For this review, take the finished solid that the model builds, in its own axes (mm). Face numbers are marked on the shaded views. A direction names the side the tool comes from. Coordinates: 2 decimals unless noted, no trailing zeros. Order: outer loops, then holes, each group sorted by start corner. A loop starts at its lowest first (then second) coordinate and runs counter-clockwise, first axis right, second up. Notation, with made-up numbers: (6.25, 7) -> (15.25, 7) arc R25 cw to (15.25, 24) -> close; hole circle Ø8 at (6.25, 60). An arc over 180 degrees is marked (long way). Return JSON: item names as keys, results as strings. Group by question number.
Item 1: Take a section at B-B (z = 0.5). Write out the cut boundary in (x, y).
Item 2: Machinability: for the marked faces 1, 2 and 3, which of the approach directions +Z, -Z, +X, -X, +Y, -Y give a long, thin tool a straight path to every point of the face, cutting with its end or side? Answer none if there is none.
Item 3: Insertion check: pin 1 (5 mm diameter, centred on y = -2, z = 13, fed in from +X); pin 2 (6 mm diameter, centred on x = -6.5, z = 19.5, fed in from -Y) (3 decimals); pin 3 (6 mm diameter, centred on x = 21, z = 15.5, fed in from -Y). Each pin has a flat end and moves straight along its axis. Give the tip position at first contact, or say it passes through.
Item 4: Draft analysis for pull direction Z (two halves, no side actions). For the marked faces 4, 5, 6 and 7, state which applies: +Z half, -Z half, draft (parallel to the pull), parting line (faces both ways), or undercut.
Item 5: Take a section at C-C (y = 13). Write out the cut boundary in (x, z), then the cut area to 3 significant figures.
Item 6: Take a section at A-A (x = 34.5). Write out the cut boundary in (y, z), then the cut area to 3 significant figures.
Item 7: For line 1 along Y through (x, z) = (34, 20.5); line 2 along Z through (x, y) = (12, -19); line 3 along Y through (x, z) = (2, 6.5) (3 decimals), list the stretches that pass through material, from the lowest coordinate up.
Item 8: Take a section at D-D (z = 18.5). Count the separate pieces of the cut face and the enclosed holes in it, then the cut area to 3 significant figures.
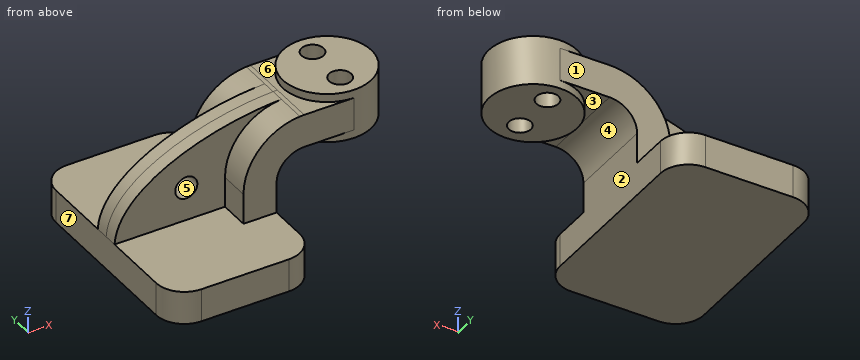
```python
from build123d import *

# Parameters (mm, degrees)
F1_DEPTH = 25
F0_W     = 10
F0_H     = 7.5
F2_DEPTH = 10
F3_DEPTH = 3.125
F5_R     = 6.35
F7_D     = 5
F9_D     = 5


with BuildPart() as f1:
    # F0 (on Front) → F1 (new body, symmetric)
    with BuildSketch(Plane.XZ):
        Polygon((8.75, 3.75), (-16.25, 3.75), (-16.25, -3.75), (16.25, -3.75), (16.25, 3.75), align=None)
    extrude(amount=F1_DEPTH, both=True)

    # F0 (on Front) → F2 (join, symmetric)
    with BuildSketch(Plane.XZ):
        with BuildLine():
            Line((8.75, 10.63), (8.75, 3.75))
            Line((8.75, 3.75), (16.25, 3.75))
            Line((16.25, 3.75), (16.25, 10.63))
            ThreePointArc((16.25, 10.63), (18.0805826176, 15.0494173824), (22.5, 16.88))
            Line((22.5, 16.88), (23.75, 16.88))
            Line((23.75, 16.88), (23.75, 24.38))
            Line((23.75, 24.38), (22.5, 24.38))
            add(Edge.make_bspline(
                [(21.5462434262, 24.3468818759), (21.8653666282, 24.3604124593), (22.1833362267, 24.3714573104), (22.5, 24.38)],
                knots=[43.0852558218, 43.0852558218, 43.0852558218, 43.0852558218, 43.8994236864, 43.8994236864, 43.8994236864, 43.8994236864], degree=3))
            ThreePointArc((21.5462434262, 24.3468818759), (12.4457309343, 20.0094548645), (8.75, 10.63))
        make_face()
        with Locations((28.75, 20.63)):
            Rectangle(F0_W, F0_H)
    extrude(amount=F2_DEPTH, both=True)

    # F0 (on Front) → F3 (join, symmetric)
    with BuildSketch(Plane.XZ):
        Polygon((8.75, 3.75), (-16.25, 3.75), (-16.25, -3.75), (16.25, -3.75), (16.25, 3.75), align=None)
        with BuildLine():
            add(Edge.make_bspline(
                [(-16.25, 3.75), (-15.4599795395, 15.953627077), (4.6584425259, 23.6308518407), (21.5462434262, 24.3468818759)],
                knots=[0, 0, 0, 0, 43.0852558218, 43.0852558218, 43.0852558218, 43.0852558218], degree=3))
            Line((-16.25, 3.75), (8.75, 3.75))
            Line((8.75, 3.75), (8.75, 10.63))
            ThreePointArc((8.75, 10.63), (12.4457309343, 20.0094548645), (21.5462434262, 24.3468818759))
        make_face()
    extrude(amount=F3_DEPTH, both=True)

    # F0 (on Front) → F4 (revolve)
    with BuildSketch(Plane.XZ):
        Polygon((33.75, 26.25), (33.75, 24.38), (33.75, 16.88), (33.75, 15), (43.75, 15), (43.75, 26.25), align=None)
    revolve(axis=Axis((33.75, 0, 20.625), (0, 0, -1)))

    # F5
    f5_edges = [f1.edges().sort_by_distance(p)[0] for p in [
        (-16.25, -25, 0),
        (16.25, -25, 0),
        (16.25, 25, 0),
        (-16.25, 25, 0),
    ]]
    fillet(f5_edges, radius=F5_R)

    # F7 (through all)
    with Locations(Plane.XY.offset(26.25)):
        with Locations((33.7088629603, 5.3247334436), (33.7088629603, -4.9510677345)):
            Hole(F7_D / 2)

    # F9 (through all)
    with Locations(Plane.XZ.offset(3.125)):
        with Locations((0, 11.303381063)):
            Hole(F9_D / 2)


solid = f1.part
```
Findings below:
{
 "1": {"outline": "(-16.25, -18.65) arc R6.35 ccw to (-9.9, -25) -> (9.9, -25) arc R6.35 ccw to (16.25, -18.65) -> (16.25, 18.65) arc R6.35 ccw to (9.9, 25) -> (-9.9, 25) arc R6.35 ccw to (-16.25, 18.65) -> close"},
 "2": {"face 1": "+Z, +X, -X, +Y", "face 2": "-Z, +X, +Y, -Y", "face 3": "-Z"},
 "3": {"pin 1": "stops at x = 43.74", "pin 2": "stops at y = -3.125", "pin 3": "stops at y = -10"},
 "4": {"face 4": "-Z half", "face 5": "undercut", "face 6": "+Z half", "face 7": "draft"},
 "5": {"outline": "(-16.25, -3.75) -> (16.25, -3.75) -> (16.25, 3.75) -> (-16.25, 3.75) -> close", "area": "244 mm2"},
 "6": {"outline": "(-9.97, 15) -> (-7.32, 15) -> (-7.32, 26.25) -> (-9.97, 26.25) -> close; (-2.58, 15) -> (2.95, 15) -> (2.95, 26.25) -> (-2.58, 26.25) -> close; (7.7, 15) -> (9.97, 15) -> (9.97, 26.25) -> (7.7, 26.25) -> close", "area": "118 mm2"},
 "7": {"line 1": "y = -10 to -7.43, -2.47 to 2.84, 7.81 to 10", "line 2": "z = -3.75 to 3.75", "line 3": "y = -3.125 to 3.125"},
 "8": {"separate pieces": "1", "enclosed holes": "2", "area": "658 mm2"}
}
